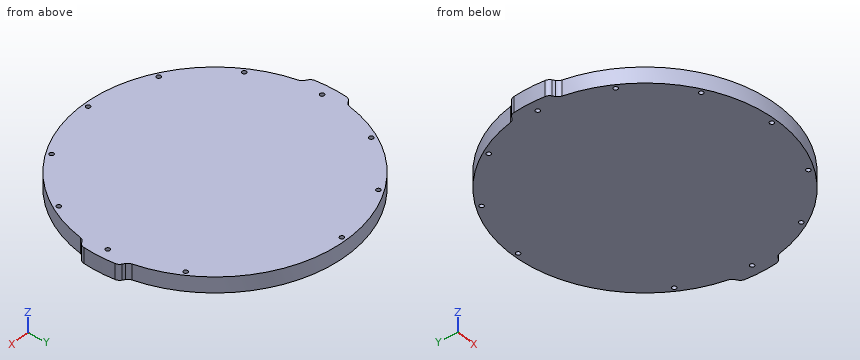
from build123d import *

# Parameters (mm, degrees)
SKETCH1_R           = 1.75
BOSS_EXTRUDE1_DEPTH = 6.35
FILLET1_R           = 5.08


with BuildPart() as part:
    # Sketch1 → Boss-Extrude1 (new, symmetric)
    with BuildSketch(Plane.XY):
        with BuildLine():
            Line((-111.997871855, 15.24), (-106.25582337, 19.05))
            ThreePointArc((-106.25582337, 19.05), (0, 107.95), (106.25582337, 19.05))
            Line((106.25582337, 19.05), (111.997871855, 15.24))
            ThreePointArc((111.997871855, 15.24), (113.03, 0), (111.997871855, -15.24))
            Line((111.997871855, -15.24), (106.25582337, -19.05))
            ThreePointArc((106.25582337, -19.05), (0, -107.95), (-106.25582337, -19.05))
            Line((-106.25582337, -19.05), (-111.997871855, -15.24))
            ThreePointArc((-111.997871855, -15.24), (-113.03, 0), (-111.997871855, 15.24))
        make_face()
        with Locations((0, 104.14)):
            Circle(SKETCH1_R, mode=Mode.SUBTRACT)
        with Locations((90.18788555, 52.07)):
            Circle(SKETCH1_R, mode=Mode.SUBTRACT)
        with Locations((104.14, 0)):
            Circle(SKETCH1_R, mode=Mode.SUBTRACT)
        with Locations((90.18788555, -52.07)):
            Circle(SKETCH1_R, mode=Mode.SUBTRACT)
        with Locations((52.07, -90.18788555)):
            Circle(SKETCH1_R, mode=Mode.SUBTRACT)
        with Locations((0, -104.14)):
            Circle(SKETCH1_R, mode=Mode.SUBTRACT)
        with Locations((-52.07, -90.18788555)):
            Circle(SKETCH1_R, mode=Mode.SUBTRACT)
        with Locations((-90.18788555, -52.07)):
            Circle(SKETCH1_R, mode=Mode.SUBTRACT)
        with Locations((-104.14, 0)):
            Circle(SKETCH1_R, mode=Mode.SUBTRACT)
        with Locations((-90.18788555, 52.07)):
            Circle(SKETCH1_R, mode=Mode.SUBTRACT)
        with Locations((-52.07, 90.18788555)):
            Circle(SKETCH1_R, mode=Mode.SUBTRACT)
    extrude(amount=BOSS_EXTRUDE1_DEPTH, both=True)

    # Fillet1
    fillet1_edges = [part.edges().sort_by_distance(p)[0] for p in [
        (-111.997871855, -15.24, 0),
        (-111.997871855, 15.24, 0),
        (-106.25582337, 19.05, 0),
        (106.25582337, 19.05, 0),
        (111.997871855, 15.24, 0),
        (111.997871855, -15.24, 0),
        (106.25582337, -19.05, 0),
        (-106.25582337, -19.05, 0),
    ]]
    fillet(fillet1_edges, radius=FILLET1_R)


solid = part.part
Can you work these out from the model? Positions are in its coordinate system, mm. Round coordinates to 2 decimals unless told otherwise and drop trailing zeros. Order: outer loops, then holes, each group sorted by start corner. A loop starts at its lowest first (then second) coordinate and runs counter-clockwise, first axis right, second up. Notation, with made-up numbers: M -26,-23 L 29,-23 A29 cw 29,1 Z; hole C 64,64 d6. An arc over 180 degrees is marked long. Use a Markdown table: item, result.
1) Imagine slicing it at B-B (x = -22.5). List the corners of the cut face in (y, z) for me.
Geometry says:
| item | result |
|---|---|
| outline | M -105.58,-6.35 L 105.58,-6.35 L 105.58,6.35 L -105.58,6.35 Z |
2) I'm going to push flat-ended pins straight in: P1, Ø4, axis at x = 90.19, y = -52.07, coming from the +Z side; P2, Ø6, axis at y = 38, z = 2, coming from the +X side; P3, Ø2, axis at y = -51.5, z = -3, coming from the -X side; P4, Ø1.5, axis at x = -1, z = -1.5, coming from the -Y side. Where does each tip first touch, or does it pass through?
Geometry says:
| item | result |
|---|---|
| P1 | stops at z = 6.35 |
| P2 | stops at x = 102.12 |
| P3 | stops at x = -95.41 |
| P4 | stops at y = -107.95 |
3) Imagine slicing it at A-A (z = -4.25). Give the number of separate pieces and of enclosed holes in the cut face, then the cut area to 3 significant figures.
Geometry says:
| item | result |
|---|---|
| separate pieces | 1 |
| enclosed holes | 11 |
| area | 36,900 mm² |
4) Imagine slicing it at C-C (y = -60.5). List the corners of the cut face in (x, z) for me, then the cut area to 3 significant figures.
Geometry says:
| item | result |
|---|---|
| outline | M -89.4,-6.35 L 89.4,-6.35 L 89.4,6.35 L -89.4,6.35 Z |
| area | 2,270 mm² |
5) If I drill on line 1 along Y through (x, z) = (-52.07, 3.75); line 2 along Y through (x, z) = (-34, 0.5); line 3 along X through (y, z) = (-3.5, 4.25), over which ranges is the centre line in solid material (lowest first)?
Geometry says:
| item | result |
|---|---|
| line 1 | y = -94.56 to -91.94, -88.44 to 88.44, 91.94 to 94.56 |
| line 2 | y = -102.46 to 102.46 |
| line 3 | x = -112.98 to 112.98 |
